Could you check a few things on this model? Use its own coordinates, in mm. A direction names the side the tool comes from. Give positions to 0.01 mm unless a question says otherwise; leave off trailing zeros. Order: outer loops, then holes, each group sorted by start corner. A loop starts at its lowest first (then second) coordinate and runs counter-clockwise, first axis right, second up. Notation, with made-up numbers: M 17,-9 L 74,-9 A36 cw 74,30 Z; hole C 89,12.25 d9. An arc over 180 degrees is marked long. Use a Markdown table: item, result. Add a question column.
Item 1: Suppose I cut it at B-B on z = 4. Write out the boundary of the cut face in (x, y).
Item 2: For faces 1 (the face through (-31.748, 7, 2)), 2 (the face through (-1, -4, 0)), 3 (the face through (26, -15, 9.5)), which set-ups out of +Z, -Z, +X, -X, +Y, -Y let a thin tool reach every point of the face, with its end or its side?
Item 3: Suppose I cut it at A-A on x = 20. Write out the boundary of the cut face in (y, z), plus the area to 4 significant figures.
Item 4: If we mould it in two halves opening along Y, with no side actions, what happens to faces 4 (the face through (-1, -20, 5)), 5 (the face through (-1, 20, 5)), 6 (the face through (-6.148, 7, 2)), 7 (the face through (35.47, -6.42, 4.82))? For each: released by +Y, released by -Y, zero draft, split by the parting line, or undercut.
Item 5: Suppose I cut it at D-D on x = -15.5. Write out the boundary of the cut face in (y, z), plus the area to 3 significant figures.
Item 6: I'm going to push flat-ended pins straight in: pin 1 Ø5.5 at (x, z) = (-16, 2) entering from +Y; pin 2 Ø4 at (x, y) = (-18.95, 7.2) entering from -Z; pin 3 Ø10 at (x, y) = (15, -3) entering from -Z. Where does each tip first touch, or does it pass through?
Item 7: If I drill on L1, parallel to Y at x = 20, z = 3.25; L2, parallel to X at y = 13, z = 2.5; L3, parallel to Y at x = 20, z = 10.15, over which ranges is the centre line in solid material (lowest first)? Write a range as from..to.
Item 8: Suppose I cut it at C-C on y = 0. Write out the boundary of the cut face in (x, z).
from build123d import *

# Parameters (mm, degrees)
F0_W      = 80
F0_H      = 40
F1_DEPTH  = 9.5
F2_R      = 16.75
F3_DEPTH  = 9.5
F4_W      = 80
F4_H      = 40
F5_DEPTH  = 1
F6_R      = 15.75
F7_DEPTH  = 1
F9_D      = 3.2639
F8_W      = 25.6
F8_H      = 25.6
F10_DEPTH = 5


with BuildPart() as f1:
    # F0 (on Top) → F1 (new body)
    with BuildSketch(Plane.XY):
        Rectangle(F0_W, F0_H)
    extrude(amount=F1_DEPTH)

    # F2 (on face) → F3 (cut)
    with BuildSketch(Plane.XY.offset(9.5)):
        with Locations((20, 0)):
            Circle(F2_R)
    extrude(amount=-F3_DEPTH, mode=Mode.SUBTRACT)

    # F4 (on face) → F5 (join)
    with BuildSketch(Plane.XY.offset(9.5)):
        Rectangle(F4_W, F4_H)
    extrude(amount=F5_DEPTH)

    # F6 (on face) → F7 (cut)
    with BuildSketch(Plane.XY.offset(10.5)):
        with Locations((20, 0)):
            Circle(F6_R)
    extrude(amount=-F7_DEPTH, mode=Mode.SUBTRACT)

    # F9 (through all)
    with Locations(Plane(origin=(0, 0, 0), x_dir=(1, 0, 0), z_dir=(0, 0, -1))):
        with Locations((-18.9480787635, -7.2)):
            Hole(F9_D / 2)

    # F8 (on face) → F10 (cut)
    with BuildSketch(Plane(origin=(0, 0, 0), x_dir=(1, 0, 0), z_dir=(0, 0, -1))):
        with Locations((-18.9480787635, -7.2)):
            Rectangle(F8_W, F8_H)
    extrude(amount=-F10_DEPTH, mode=Mode.SUBTRACT)


solid = f1.part
Findings below:
| question | item | result |
|---|---|---|
| 1 | outline | M -40,-20 L 40,-20 L 40,20 L -6.15,20 L -6.15,-5.6 L -31.75,-5.6 L -31.75,20 L -40,20 Z; hole C 20,0 d33.5 |
| 2 | face 1 | -Z, +Y |
| 2 | face 2 | -Z, +X, -X, +Y, -Y |
| 2 | face 3 | -Z |
| 3 | outline | M -20,0 L -16.75,0 L -16.75,9.5 L -15.75,9.5 L -15.75,10.5 L -20,10.5 Z; M 15.75,9.5 L 16.75,9.5 L 16.75,0 L 20,0 L 20,10.5 L 15.75,10.5 Z |
| 3 | area | 70.25 mm^2 |
| 4 | face 4 | released by -Y |
| 4 | face 5 | released by +Y |
| 4 | face 6 | zero draft |
| 4 | face 7 | undercut |
| 5 | outline | M -20,0 L -5.6,0 L -5.6,5 L 20,5 L 20,10.5 L -20,10.5 Z |
| 5 | area | 292 mm^2 |
| 6 | pin 1 | stops at y = -5.6 |
| 6 | pin 2 | stops at z = 5 |
| 6 | pin 3 | passes through |
| 7 | L1 | y = -20..-16.75, 16.75..20 |
| 7 | L2 | x = -40..-31.75, -6.15..9.44, 30.56..40 |
| 7 | L3 | y = -20..-15.75, 15.75..20 |
| 8 | outline | M -40,0 L -31.75,0 L -31.75,5 L -6.15,5 L -6.15,0 L 3.25,0 L 3.25,9.5 L 4.25,9.5 L 4.25,10.5 L -40,10.5 Z; M 35.75,9.5 L 36.75,9.5 L 36.75,0 L 40,0 L 40,10.5 L 35.75,10.5 Z |
